Source: CAD feature listing. Evaluate the final solid. Frame: model axes, mm. Coordinates: 2 decimals unless noted, no trailing zeros. Loops run counter-clockwise (first coordinate to the right, second up) from the corner with the lowest first, then second, coordinate; pieces in that order, holes last. Notation, with made-up numbers: (0.5, 74) -> (53.5, 74) arc R25 cw to (53.5, 87) -> close; hole circle Ø5 at (67.25, -2). An arc over 180 degrees is marked (long way). Answer as a JSON object with one key per item and string values. Group by question number.
from build123d import *

# Parameters (mm, degrees)
F0_W     = 100
F0_H     = 100
F1_DEPTH = 100
F3_R     = 1.2
F4_R     = 33.33333
F5_DEPTH = 100.001


with BuildPart() as f1:
    # F0 (on Top) → F1 (new body)
    with BuildSketch(Plane.XY):
        Rectangle(F0_W, F0_H)
    extrude(amount=F1_DEPTH)

    # F3
    f3_edges = [f1.edges().sort_by_distance(p)[0] for p in [
        (-50, 0, 100),
        (0, 50, 100),
        (50, 0, 100),
        (0, -50, 100),
        (-50, -50, 50),
        (-50, 50, 50),
        (50, -50, 50),
        (50, 50, 50),
        (50, 0, 0),
        (0, -50, 0),
        (-50, 0, 0),
        (0, 50, 0),
    ]]
    fillet(f3_edges, radius=F3_R)

    # F4 (on face) → F5 (cut, through all)
    with BuildSketch(Plane.YZ.offset(50)):
        with Locations((0, 50)):
            Circle(F4_R)
    extrude(amount=-F5_DEPTH, mode=Mode.SUBTRACT)


solid = f1.part
1. Section query A-A on y = 0. Return loops of the section in (x, z).
2. Section query C-C on x = -16.5. Return loops of the section in (y, z), then the cut area to 3 significant figures.
3. Section query B-B on z = 50. Return loops of the section in (x, y).
4. Mould query, pull axis Z, two halves, no side actions, for faces 1 (the face through (-1, 1, 0)), 2 (the face through (0.7, -4.34, 83.05)), 3 (the face through (50, 10, 82)). Classes: pulls with the +Z half, pulls with the -Z half, needs draft (parallel to the pull), parting line crosses it, or undercut.
5. Ray query, L1, parallel to Z at x = 0.5, y = 0; L2, parallel to Y at x = 40, z = 27; L3, parallel to Z at x = -27, y = -13.5. Return the intervals inside material, ascending.
Solved:
{
 "1": {"outline": "(-50, 1.2) arc R1.2 ccw to (-48.8, 0) -> (48.8, 0) arc R1.2 ccw to (50, 1.2) -> (50, 16.67) -> (-50, 16.67) -> close; (-50, 83.33) -> (50, 83.33) -> (50, 98.8) arc R1.2 ccw to (48.8, 100) -> (-48.8, 100) arc R1.2 ccw to (-50, 98.8) -> close"},
 "2": {"outline": "(-50, 1.2) arc R1.2 ccw to (-48.8, 0) -> (48.8, 0) arc R1.2 ccw to (50, 1.2) -> (50, 98.8) arc R1.2 ccw to (48.8, 100) -> (-48.8, 100) arc R1.2 ccw to (-50, 98.8) -> close; hole circle Ø66.67 at (0, 50)", "area": "6,510 mm^2"},
 "3": {"outline": "(-50, -48.8) arc R1.2 ccw to (-48.8, -50) -> (48.8, -50) arc R1.2 ccw to (50, -48.8) -> (50, -33.33) -> (-50, -33.33) -> close; (-50, 33.33) -> (50, 33.33) -> (50, 48.8) arc R1.2 ccw to (48.8, 50) -> (-48.8, 50) arc R1.2 ccw to (-50, 48.8) -> close"},
 "4": {"face 1": "pulls with the -Z half", "face 2": "undercut", "face 3": "needs draft"},
 "5": {"L1": "0 to 16.67, 83.33 to 100", "L2": "-50 to -24.13, 24.13 to 50", "L3": "0 to 19.52, 80.48 to 100"}
}
